Geometry: final body of the model. Coordinates: model frame, mm. A direction names the side the tool comes from. Give positions to 0.01 mm unless a question says otherwise; leave off trailing zeros. Loops run counter-clockwise (first coordinate to the right, second up) from the corner with the lowest first, then second, coordinate; pieces in that order, holes last.
Autodesk Inventor part; units mm, degrees
ref_plane "YZ Plane" through (0, 0, 0) normal (1, 0, 0) x (0, 1, 0)
ref_plane "XZ Plane" through (0, 0, 0) normal (0, 1, 0) x (-1, 0, 0)
ref_plane "XY Plane" through (0, 0, 0) normal (0, 0, 1) x (1, 0, 0)
sketch "Sketch1" plane through (0, 0, 0) normal (0, 0, 1) x (1, 0, 0)
  line L0 (0, 0) -> (37.5, 0)
  line L1 (37.5, 0) -> (37.5, 24.5)
  line L2 (37.5, 24.5) -> (0, 24.5)
  line L3 (0, 24.5) -> (0, 0)
  dimension "d0" = 37.5
  dimension "d1" = 24.5
extrude "Extrusion1" add sketch "Sketch1" along normal blind 11.5
sketch "Sketch2" plane through (0, 0, 0) normal (-1, 0, 0) x (0, 0, 1)
  line L0 (11.5, 24.5) -> (11.5, 0)
  line L1 (0, 24.5) -> (11.5, 24.5)
  circle A0 centre (12, 14.5) radius 4.1
  dimension "d4" = 8.2
  dimension "d5" = 0.5
  dimension "d6" = 10
extrude "Extrusion2" cut sketch "Sketch2" against normal up to surface (37.5 mm away)
sketch "Sketch3" plane through (0, 0, 0) normal (0, 0, -1) x (-1, 0, 0)
  line L0 (0, 24.5) -> (0, 0)
  line L1 (0, 18.5694) -> (0, 10.4306)
  line L2 (0, 0) -> (-37.5, 0)
  point P0 (-6, 21)
  point P1 (-32, 21)
  point P2 (-32, 4.5)
  point P3 (-6, 4.5)
  dimension "d9" = 6
  dimension "d10" = 32
  dimension "d30" = 4.5
  dimension "d32" = 21
hole "Hole1" at (6, 21, 0) at (32, 21, 0) at (32, 4.5, 0) at (6, 4.5, 0) direction (0, 0, 1) diameter 4.5 depth 11.5 counterbore diameter 8 counterbore depth 4
properties part number "YMotorCapLeft" material "ABS Plastic"
Item 1: Section query B-B on z = 5.5. Return loops of the section in (x, y), plus the area to 3 significant figures.
Values follow:
outline: (0, 0) - (37.5, 0) - (37.5, 24.5) - (0, 24.5) - close; hole circle Ø4.5 at (6, 4.5); hole circle Ø4.5 at (6, 21); hole circle Ø4.5 at (32, 4.5); hole circle Ø4.5 at (32, 21)
area: 855 mm2
Item 2: Set-up query: faces 4 (the face through (34, 6, 4)), 5 (the face through (5.324, 6.646, 7.802)). Return all of +Z, -Z, +X, -X, +Y, -Y with unobstructed straight access to the full face (end or side cutting, diameter ignored); none if empty.
Values follow:
face 4: -Z
face 5: +Z, -Z
Item 3: Section query D-D on x = 21.5. Return loops of the section in (y, z).
Values follow:
outline: (0, 0) - (24.5, 0) - (24.5, 11.5) - (18.57, 11.5) arc R4.1 cw to (10.43, 11.5) - (0, 11.5) - close
Item 4: Pin query (flat end, axial travel): pin 1 (7 mm diameter, centred on x = 6, y = 4.5, fed in from -Z). Return the tip coordinate at first contact, or that it passes through.
Values follow:
pin 1: stops at z = 4
Item 5: Section query C-C on y = 21. Return loops of the section in (x, z), plus the area to 3 significant figures.
Values follow:
outline: (0, 0) - (2, 0) - (2, 4) - (3.75, 4) - (3.75, 11.5) - (0, 11.5) - close; (8.25, 4) - (10, 4) - (10, 0) - (28, 0) - (28, 4) - (29.75, 4) - (29.75, 11.5) - (8.25, 11.5) - close; (34.25, 4) - (36, 4) - (36, 0) - (37.5, 0) - (37.5, 11.5) - (34.25, 11.5) - close
area: 300 mm2
Item 6: Draft query along Y for faces 1 (the face through (18, 22, 11.5)), 2 (the face through (5.324, 23.146, 7.802)), 3 (the face through (18, 0, 6)). Return one class per face: +Y half, -Y half, draft (parallel to the pull), parting line (faces both ways), or undercut.
Values follow:
face 1: draft
face 2: undercut
face 3: -Y half
Item 7: Ray query, probe 1 along X at (y, z) = (21, 1.4); probe 2 along X at (y, z) = (21, 9); probe 3 along Y at (x, z) = (6, 6). Return the intervals inside material, ascending.
Values follow:
probe 1: x = 0 to 2, 10 to 28, 36 to 37.5
probe 2: x = 0 to 3.75, 8.25 to 29.75, 34.25 to 37.5
probe 3: y = 0 to 2.25, 6.75 to 18.75, 23.25 to 24.5
Item 8: Section query A-A on x = 6. Return loops of the section in (y, z), plus the area to 3 significant figures.
Values follow:
outline: (0, 0) - (0.5, 0) - (0.5, 4) - (2.25, 4) - (2.25, 11.5) - (0, 11.5) - close; (6.75, 4) - (8.5, 4) - (8.5, 0) - (17, 0) - (17, 4) - (18.75, 4) - (18.75, 11.5) - (18.57, 11.5) arc R4.1 cw to (10.43, 11.5) - (6.75, 11.5) - close; (23.25, 4) - (24.5, 4) - (24.5, 11.5) - (23.25, 11.5) - close
area: 130 mm2
